The listing builds one solid part. Answer for the finished solid, in the listing's coordinates (mm). Face numbers are marked on the shaded views. A direction names the side the tool comes from. Coordinates: 2 decimals unless noted, no trailing zeros. Write each loop counter-clockwise with the first axis right and the second up, starting at its lowest first coordinate (ties: lowest second). Pieces come first, ordered by that corner, then holes.
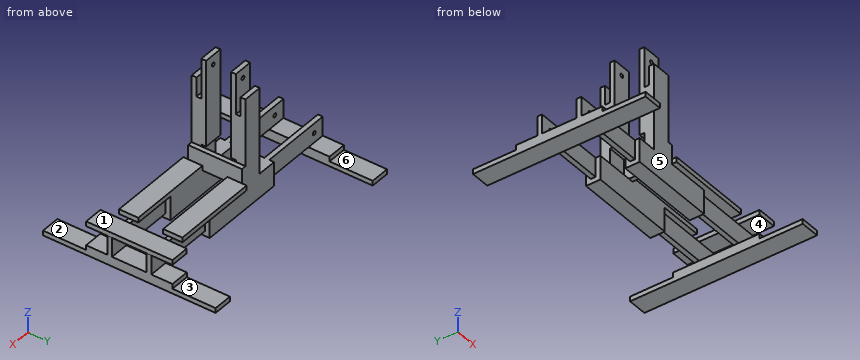
from build123d import *

# Parameters (mm, degrees)
F0_W      = 304.8
F0_H      = 25.4
F1_DEPTH  = 6.35
F2_W      = 114.3
F2_H      = 25.4
F3_DEPTH  = 6.35
F4_W      = 114.3
F4_H      = 25.4
F5_DEPTH  = 6.35
F7_D      = 5.08
F8_W      = 114.3
F8_H      = 19.05
F9_DEPTH  = 6.35
F10_W     = 25.4
F10_H     = 57.15
F11_DEPTH = 6.35
F12_W     = 25.4
F12_H     = 114.3
F13_DEPTH = 6.35
F14_W     = 25.4
F14_H     = 57.15
F15_DEPTH = 6.35
F16_W     = 25.4
F16_H     = 114.3
F17_DEPTH = 6.35
F18_W     = 25.4
F18_H     = 57.15
F19_DEPTH = 6.35
F20_W     = 6.35
F20_H     = 57.15
F21_DEPTH = 25.4
F22_W     = 114.3
F22_H     = 25.4
F23_DEPTH = 6.35
F24_W     = 25.4
F24_H     = 6.35
F25_DEPTH = 88.9
F26_W     = 25.4
F26_H     = 6.35
F27_DEPTH = 114.3
F28_W     = 25.4
F28_H     = 114.3
F29_DEPTH = 6.35
F31_D     = 5.08


with BuildPart() as f1:
    # F0 (on Front) → F1 (new body)
    with BuildSketch(Plane.XZ):
        with Locations((9.459311, -15.122586)):
            Rectangle(F0_W, F0_H)
    extrude(amount=F1_DEPTH)

    # F2 (on face) → F3 (join)
    with BuildSketch(Plane.XZ.offset(6.35)):
        with Locations((9.459311, -15.122586)):
            Rectangle(F2_W, F2_H)
    extrude(amount=F3_DEPTH)

    # F4 (on face) → F5 (join)
    with BuildSketch(Plane(origin=(0, 0, 0), x_dir=(-1, 0, 0), z_dir=(0, 1, 0))):
        with Locations((-9.459311, -15.122586)):
            Rectangle(F4_W, F4_H)
    extrude(amount=F5_DEPTH)

    # F7 (through all)
    with Locations(Plane.XZ.offset(6.35)):
        with Locations((-127.700689, -15.122586)):
            Hole(F7_D / 2)

    # F8 (on face) → F9 (join)
    with BuildSketch(Plane(origin=(0, 0, -27.822586), x_dir=(1, 0, 0), z_dir=(0, 0, -1))):
        with Locations((9.459311, 3.175)):
            Rectangle(F8_W, F8_H)
    extrude(amount=F9_DEPTH)

    # F10 (on face) → F11 (join)
    with BuildSketch(Plane(origin=(0, 0, -27.822586), x_dir=(1, 0, 0), z_dir=(0, 0, -1))):
        with Locations((-130.240689, 0.635)):
            Rectangle(F10_W, F10_H)
    extrude(amount=F11_DEPTH)

    # F12 (on face) → F13 (join)
    with BuildSketch(Plane(origin=(0, 0, -34.172586), x_dir=(1, 0, 0), z_dir=(0, 0, -1))):
        with Locations((-130.240689, -27.94)):
            Rectangle(F12_W, F12_H)
    extrude(amount=F13_DEPTH)

    # F14 (on face) → F15 (join)
    with BuildSketch(Plane(origin=(0, 0, -27.822586), x_dir=(1, 0, 0), z_dir=(0, 0, -1))):
        with Locations((149.159311, 0.635)):
            Rectangle(F14_W, F14_H)
    extrude(amount=F15_DEPTH)

    # F16 (on face) → F17 (join)
    with BuildSketch(Plane(origin=(0, 0, -34.172586), x_dir=(1, 0, 0), z_dir=(0, 0, -1))):
        with Locations((149.159311, -27.94)):
            Rectangle(F16_W, F16_H)
    extrude(amount=F17_DEPTH)

    # F18 (on face) → F19 (join)
    with BuildSketch(Plane.XY.offset(-2.422586)):
        with Locations((149.190135, -0.635)):
            Rectangle(F18_W, F18_H)
    extrude(amount=F19_DEPTH)

    # F20 (on face) → F21 (join)
    with BuildSketch(Plane.XY.offset(-2.422586)):
        with Locations((6.284311, -22.225)):
            Rectangle(F20_W, F20_H)
    extrude(amount=F21_DEPTH)

    # F22 (on face) → F23 (join)
    with BuildSketch(Plane.XY.offset(-2.422586)):
        with Locations((66.609311, 0)):
            Rectangle(F22_W, F22_H)
    extrude(amount=F23_DEPTH)

    # F24 (on face) → F25 (join)
    with BuildSketch(Plane.XY.offset(-2.422586)):
        with Locations((-9.590689, -3.175)):
            Rectangle(F24_W, F24_H)
    extrude(amount=F25_DEPTH)

    # F26 (on face) → F27 (join)
    with BuildSketch(Plane.XY.offset(-2.422586)):
        with Locations((-9.590689, 3.175)):
            Rectangle(F26_W, F26_H)
    extrude(amount=F27_DEPTH)

    # F28 (on face) → F29 (join)
    with BuildSketch(Plane.XZ.offset(6.35)):
        with Locations((-9.590689, 82.667414)):
            Rectangle(F28_W, F28_H)
    extrude(amount=F29_DEPTH)

    # F31 (through all)
    with Locations(Plane(origin=(0, -6.35, 0), x_dir=(-1, 0, 0), z_dir=(0, 1, 0))):
        with Locations((9.590689, 127.117414)):
            Hole(F31_D / 2)

    # F32: F1 across face


with BuildPart() as f1_1:
    add(f1.part)
    add(f1.part.mirror(Plane(origin=(-130.240689, -29.21, -34.172586), x_dir=(1, 0, 0), z_dir=(0, -1, 0))))


solid = f1_1.part
Q1. The part is cut by section B-B, the plane y = 31.5. Write down the section's boundary in (x, z), then the cut area to 3 significant figures.
Answers below:
outline: (-142.94, -40.52) - (-117.54, -40.52) - (-117.54, -34.17) - (-142.94, -34.17) - close; (136.46, -40.52) - (161.86, -40.52) - (161.86, -34.17) - (136.46, -34.17) - close
area: 323 mm2
Q2. The part is cut by section A-A, the plane x = -69.5. Write down the section's boundary in (y, z), then the cut area to 3 significant figures.
Answers below:
outline: (-58.42, -27.82) - (-52.07, -27.82) - (-52.07, -2.42) - (-58.42, -2.42) - close; (-6.35, -27.82) - (0, -27.82) - (0, -2.42) - (-6.35, -2.42) - close
area: 323 mm2
Q3. Which of the six approach directions +Z, -Z, +X, -X, +Y, -Y give full straight-line access (tool end or side, diameter ignored) to the marked faces 1, 2 and 3?
Answers below:
face 1: +Z, +X, +Y, -Y
face 2: +Z, +X, -X, -Y
face 3: +Z, +X, -X, +Y
Q4. Determine the mould class of the marked faces 4, 5 and 6 for opening direction Y: released by +Y, released by -Y, zero draft, split by the parting line, or undercut.
Answers below:
face 4: undercut
face 5: released by -Y
face 6: zero draft
Q5. Find the intervals of material crossed by probe 1 along Y at (x, z) = (58, -7.5); probe 2 along Y at (x, z) = (129, -4); probe 3 along X at (y, z) = (-9, 101), in increasing order.
Answers below:
probe 1: y = -64.77 to -45.72, -12.7 to 6.35
probe 2: y = -58.42 to -52.07, -6.35 to 0
probe 3: x = -22.29 to 3.11
Q6. Given pin 1 (1.9 mm diameter, centred on x = 128.5, y = -4, fed in from +Z); pin 2 (3 mm diameter, centred on x = 6, z = -4.5, fed in from -Y); pin 3 (20.5 mm diameter, centred on x = -14.5, z = 118.5, fed in from +Y); pin 4 (4.5 mm diameter, centred on x = -9.59, z = 127.12, fed in from +Y), each flat-ended and moving along its own axis, determine where each tip first touches the part or whether it passes through.
Answers below:
pin 1: stops at z = -2.42
pin 2: stops at y = -64.77
pin 3: stops at y = 6.35
pin 4: passes through
Q7. The part is cut by section C-C, the plane z = 97.5. Write down the section's boundary in (x, y), then the cut area to 3 significant figures.
Answers below:
outline: (-22.29, -64.77) - (3.11, -64.77) - (3.11, -58.42) - (-22.29, -58.42) - close; (-22.29, -52.07) - (3.11, -52.07) - (3.11, -45.72) - (-22.29, -45.72) - close; (-22.29, -12.7) - (3.11, -12.7) - (3.11, -6.35) - (-22.29, -6.35) - close; (-22.29, 0) - (3.11, 0) - (3.11, 6.35) - (-22.29, 6.35) - close
area: 645 mm2
Q8. The part is cut by section D-D, the plane y = -40. Write down the section's boundary in (x, z).
Answers below:
outline: (-142.94, -40.52) - (-117.54, -40.52) - (-117.54, -27.82) - (-142.94, -27.82) - close; (3.11, -2.42) - (9.46, -2.42) - (9.46, 22.98) - (3.11, 22.98) - close; (136.46, -40.52) - (161.86, -40.52) - (161.86, -27.82) - (136.46, -27.82) - close; (136.49, -2.42) - (161.89, -2.42) - (161.89, 3.93) - (136.49, 3.93) - close
